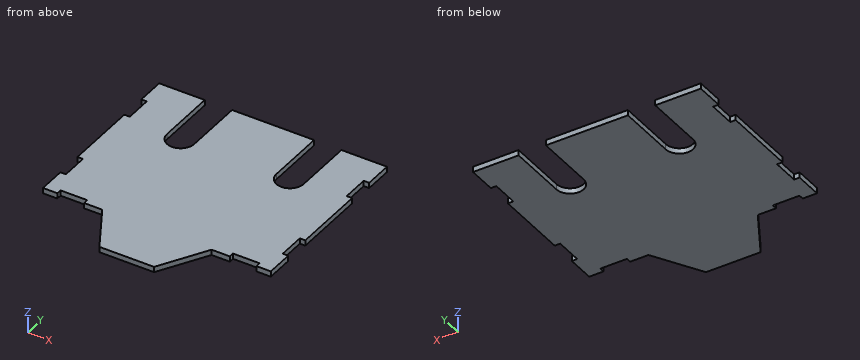
```python
from build123d import *

# Parameters (mm, degrees)
EXTRUDE_1_DEPTH = 6


with BuildPart() as part:
    # Эскиз1 → Бобышка-Вытянуть1 (new body)
    with BuildSketch(Plane.XY):
        with BuildLine():
            Line((0, 0), (-50, 0))
            Line((-50, 0), (-50, -65))
            ThreePointArc((-50, -65), (-65, -80), (-80, -65))
            Line((-80, -65), (-80, 0))
            Line((-80, 0), (-170, 0))
            Line((-170, 0), (-170, -65))
            ThreePointArc((-170, -65), (-185, -80), (-200, -65))
            Line((-200, -65), (-200, 0))
            Line((-200, 0), (-250, 0))
            Line((-250, 0), (-250, -30.7))
            Line((-250, -30.7), (-244, -30.7))
            Line((-244, -30.7), (-244, -60))
            Line((-244, -60), (-250, -60))
            Line((-250, -60), (-250, -140.7))
            Line((-250, -140.7), (-244, -140.7))
            Line((-244, -140.7), (-244, -170))
            Line((-244, -170), (-250, -170))
            Line((-250, -170), (-250, -200))
            Line((-250, -200), (-234.3, -200))
            Line((-234.3, -200), (-234.3, -194.55))
            Line((-234.3, -194.55), (-205, -194.55))
            Line((-205, -194.55), (-205, -200))
            Line((-205, -200), (-185, -200))
            Line((-185, -200), (-155, -251.961524227))
            Line((-155, -251.961524227), (-95, -251.961524227))
            Line((-95, -251.961524227), (-65, -200))
            Line((-65, -200), (-45, -200))
            Line((-45, -200), (-45, -194.55))
            Line((-45, -194.55), (-15.7, -194.55))
            Line((-15.7, -194.55), (-15.7, -200))
            Line((-15.7, -200), (0, -200))
            Line((0, -200), (0, -170))
            Line((0, -170), (-6, -170))
            Line((-6, -170), (-6, -140.7))
            Line((-6, -140.7), (0, -140.7))
            Line((0, -140.7), (0, -60))
            Line((0, -60), (-6, -60))
            Line((-6, -60), (-6, -30.7))
            Line((-6, -30.7), (0, -30.7))
            Line((0, -30.7), (0, 0))
        make_face()
    extrude(amount=EXTRUDE_1_DEPTH)


solid = part.part
```
Input: part model. Units: mm. Frame: model coordinates. Give positions to 0.01 mm unless a question says otherwise; leave off trailing zeros. Write each loop counter-clockwise with the first axis right and the second up, starting at its lowest first coordinate (ties: lowest second). Pieces come first, ordered by that corner, then holes. Notation, with made-up numbers: (40, 23) - (96, 23) arc R26 cw to (96, 50) - close; hole circle Ø10 at (72.25, 57). An arc over 180 degrees is marked (long way). Write item = value, one per line. Start each with the question number.
1. Section query B-B, the plane x = -73.5. Output: boundary loops of the cut face in (y, z).
2. First-contact query: pin 1 Ø3 at (y, z) = (-44.5, 3.5) entering from +X; pin 2 Ø3 at (x, z) = (-2, 1.5) entering from -Y. Flat tips, straight axial feed; report the tip coordinate or a pass-through.
3. Section query A-A, the plane y = -44. Output: boundary loops of the cut face in (x, z).
4. Section query C-C, the plane y = -149. Output: boundary loops of the cut face in (x, z).
5. Ray query, L1, parallel to X at y = -198, z = 3.9; L2, parallel to X at y = -30.5, z = 0.4; L3, parallel to X at y = -160.5, z = 5.5. Return the intervals inside material, ascending.
Check sheet entries:
q1.outline = (-214.72, 0) - (-77.36, 0) - (-77.36, 6) - (-214.72, 6) - close
q2.pin_1 = -6
q2.pin_2 = -200
q3.outline = (-244, 0) - (-200, 0) - (-200, 6) - (-244, 6) - close; (-170, 0) - (-80, 0) - (-80, 6) - (-170, 6) - close; (-50, 0) - (-6, 0) - (-6, 6) - (-50, 6) - close
q4.outline = (-244, 0) - (-6, 0) - (-6, 6) - (-244, 6) - close
q5.L1 = -250 to -234.3, -205 to -45, -15.7 to 0
q5.L2 = -250 to -200, -170 to -80, -50 to 0
q5.L3 = -244 to -6
